from build123d import *

# Parameters (mm, degrees)
SKETCH1_R               = 6.35
EXTRUDE1_DEPTH          = 5.55625
SKETCH7_OUTSIDE_W       = 115.268
SKETCH7_OUTSIDE_H       = 118.216
SKETCH7_OUTSIDE_R       = 9.525
EXTRUDE2_DEPTH          = 25.4
EXTRUDE2_DRAFT          = -60
MIRROR1_COPY_1_SKETCH_W = 115.268
MIRROR1_COPY_1_SKETCH_H = 118.216
MIRROR1_COPY_1_SKETCH_R = 9.525
MIRROR1_COPY_1_DEPTH    = 25.4
MIRROR1_COPY_1_DRAFT    = -60


with BuildPart() as part:
    # Sketch1 → Extrude1 (new, symmetric)
    with BuildSketch(Plane.XY):
        Polygon((-9.525, 5.499261314), (-9.525, -5.499261314), (0, -10.998522628), (9.525, -5.499261314), (9.525, 5.499261314), (0, 10.998522628), align=None)
        Circle(SKETCH1_R, mode=Mode.SUBTRACT)
    extrude(amount=EXTRUDE1_DEPTH, both=True)


with BuildPart() as extrude2_tool:
    # Sketch7 outside → Extrude2 (with draft: the straight prism first)
    with BuildSketch(Plane.XY.offset(5.55625)):
        Rectangle(SKETCH7_OUTSIDE_W, SKETCH7_OUTSIDE_H)
        Circle(SKETCH7_OUTSIDE_R, mode=Mode.SUBTRACT)
    extrude(amount=-EXTRUDE2_DEPTH)
    # Extrude2: the draft: its side faces are tilted about the plane it starts from
    extrude2_sides = [extrude2_tool.faces().sort_by_distance(p)[0] for p in [
        (0, -59.108, -7.14375),
        (57.634, 0, -7.14375),
        (0, 59.108, -7.14375),
        (-57.634, 0, -7.14375),
        (-9.525, 0, -7.14375),
    ]]
    draft(extrude2_sides, Plane.XY.offset(5.55625), EXTRUDE2_DRAFT)


with BuildPart() as part_1:
    add(part.part)

    # Extrude2: cut by extrude2_tool
    add(extrude2_tool.part, mode=Mode.SUBTRACT)


with BuildPart() as mirror1_copy_1_tool:
    # Mirror1 copy 1 sketch → Mirror1 copy 1 (with draft: the straight prism first)
    with BuildSketch(Plane(origin=(0, 0, -5.55625), x_dir=(1, 0, 0), z_dir=(0, 0, -1))):
        Rectangle(MIRROR1_COPY_1_SKETCH_W, MIRROR1_COPY_1_SKETCH_H)
        Circle(MIRROR1_COPY_1_SKETCH_R, mode=Mode.SUBTRACT)
    extrude(amount=-MIRROR1_COPY_1_DEPTH)
    # Mirror1 copy 1: the draft: its side faces are tilted about the plane it starts from
    mirror1_copy_1_sides = [mirror1_copy_1_tool.faces().sort_by_distance(p)[0] for p in [
        (0, -59.108, 7.14375),
        (57.634, 0, 7.14375),
        (0, 59.108, 7.14375),
        (-57.634, 0, 7.14375),
        (-9.525, 0, 7.14375),
    ]]
    draft(mirror1_copy_1_sides, Plane(origin=(0, 0, -5.55625), x_dir=(1, 0, 0), z_dir=(0, 0, -1)), MIRROR1_COPY_1_DRAFT)


with BuildPart() as part_2:
    add(part_1.part)

    # Mirror1 copy 1: cut by mirror1_copy_1_tool
    add(mirror1_copy_1_tool.part, mode=Mode.SUBTRACT)


solid = part_2.part
The model under review builds one solid part; all positions refer to its coordinate system, in mm. Coordinates: 2 decimals unless noted, no trailing zeros. Write each loop counter-clockwise with the first axis right and the second up, starting at its lowest first coordinate (ties: lowest second). Pieces come first, ordered by that corner, then holes. Notation, with made-up numbers: (17, 60.5) - (76, 60.5) arc R15 cw to (76, 82.5) - close; hole circle Ø10 at (19, 17.25). An arc over 180 degrees is marked (long way). Answer as CSV lines item,"result".
(1) Clearance check with a flat-ended pin moving along its axis: pin 1 Ø1.5 at (x, y) = (-3.5, 3) entering from +Z. State where the tip first meets the part, or that it passes through.
Data:
pin 1,"passes through"
(2) We need section A-A (z = 0.5). Give the boundary of the cut face in (x, y) (3 decimals).
Data:
outline,"(-9.525, -5.499) - (0, -10.999) - (9.525, -5.499) - (9.525, 5.499) - (0, 10.999) - (-9.525, 5.499) - close; hole circle Ø12.7 at (0, 0)"
(3) For line 1 along Y through (x, z) = (-2.5, -2.5); line 2 along Y through (x, z) = (-1.25, 1.75); line 3 along X through (y, z) = (3.5, -1.5) (3 decimals), list the stretches that pass through material, from the lowest coordinate up. Write a range as [from, to].
Data:
line 1,"y = [-9.56, -5.84], [5.84, 9.56]"
line 2,"y = [-10.28, -6.23], [6.23, 10.28]"
line 3,"x = [-9.525, -5.298], [5.298, 9.525]"
(4) Mouldability with a two-part tool opening along X and no side actions: class faces 1 (the flat face through (9.525, 0, 0)), 2 (the cylindrical face through (-1.38, -6.2, -0.08)), 3 (the flat face through (6.2, -2, -5.556)), 4 (the flat face through (-9.525, 0, 0)) as pulls with the +X half, pulls with the -X half, needs draft (parallel to the pull), parting line crosses it, or undercut.
Data:
face 1,"pulls with the +X half"
face 2,"undercut"
face 3,"needs draft"
face 4,"pulls with the -X half"
